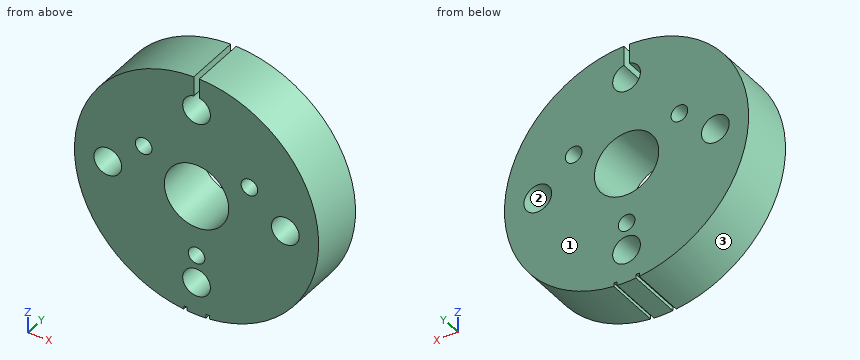
Autodesk Inventor part; units mm, degrees
ref_plane "YZ Plane" through (0, 0, 0) normal (1, 0, 0) x (0, 1, 0)
ref_plane "XZ Plane" through (0, 0, 0) normal (0, 1, 0) x (-1, 0, 0)
ref_plane "XY Plane" through (0, 0, 0) normal (0, 0, 1) x (1, 0, 0)
sketch "Эскиз1" plane through (0, 0, 0) normal (0, 1, 0) x (-1, 0, 0)
  arc A0 (-0.25, 9.2247) -> (0.25, 9.2247) centre (0, 8) ccw
  line L0 (-0.25, 10.9972) -> (-0.25, 9.2247)
  arc A1 (-0.25, 10.9972) -> (-1.1469, -10.94) centre (0, 0) ccw
  line L1 (-1.1469, -10.6297) -> (-1.1469, -10.94)
  line L2 (-0.8473, -10.6297) -> (-1.1469, -10.6297)
  line L3 (-0.8473, -10.9673) -> (-0.8473, -10.6297)
  arc A2 (-0.8473, -10.9673) -> (0.8535, -10.9668) centre (0, 0) ccw
  line L4 (0.8535, -10.6297) -> (0.8535, -10.9668)
  line L5 (1.1541, -10.6297) -> (0.8535, -10.6297)
  line L6 (1.1541, -10.9393) -> (1.1541, -10.6297)
  arc A3 (1.1541, -10.9393) -> (0.25, 10.9972) centre (0, 0) ccw
  line L7 (0.25, 9.2247) -> (0.25, 10.9972)
  circle A4 centre (8, 0) radius 1.25
  circle A5 centre (0, -8) radius 1.25
  circle A6 centre (-8, 0) radius 1.25
  circle A7 centre (0, -5.5) radius 0.75
  circle A8 centre (4.7631, 2.75) radius 0.75
  circle A9 centre (-4.7631, 2.75) radius 0.75
  circle A10 centre (0, 0) radius 2.9
  arc A11 (0.25, 9.2247) -> (-0.25, 9.2247) centre (0, 8) ccw
extrude "Выдавливание1" add sketch "Эскиз1" along normal blind 5 contours A0 L7 A3 L6 L5 L4 A2 L3 L2 L1 A1 L0
properties part number "проставка"
Could you check a few things on this model? Use its own coordinates, in mm. Face numbers are marked on the shaded views. Coordinates: 2 decimals unless noted, no trailing zeros. Write each loop counter-clockwise with the first axis right and the second up, starting at its lowest first coordinate (ties: lowest second). Pieces come first, ordered by that corner, then holes. Notation, with made-up numbers: M 65.5,24 L 116.5,24 A17 ccw 116.5,44 Z; hole C 1.25,-31.5 d11. An arc over 180 degrees is marked long. Answer as CSV lines item,"result". Start each with the question number.
1) I want a section at A-A, the plane x = -1.75. Please give me the cut outline in (y, z).
2) I want a section at C-C, the plane y = 2.25. Please give me the cut outline in (x, z).
3) I want a section at B-B, the plane z = 9.5. Please give me the cut outline in (x, y).
4) Please list where these lines run through material, in increasing order: line 1 (Z direction, x = 0, y = 2.3); line 2 (X direction, y = 4.5, z = 3.25); line 3 (Z direction, x = 8, y = 4.05). Write a range as from..to.
5) For P1, Ø2, axis at y = 4, z = -2.5, coming from the -X side; P2, Ø1.4, axis at x = -4.76, z = 2.75, coming from the -Y side; P3, Ø1, axis at x = 1.5, y = 3.5, coming from the -Z side; P4, Ø0.9, axis at y = 3.5, z = 10, coming from the -X side, each with a flat end and sliding along its axis, tell me the tip position at first contact or that it passes through.
6) We'd pull the mould along X, two halves only. Please class the marked faces 1, 2 and 3: +X half, -X half, draft (parallel to the pull), parting line (faces both ways), or undercut.
7) I want a section at D-D, the plane z = 5. Please give me the cut outline in (x, y), and give its area (3 significant figures).
Data:
1,outline,"M 0,-10.86 L 5,-10.86 L 5,-2.31 L 0,-2.31 Z; M 0,2.31 L 5,2.31 L 5,10.86 L 0,10.86 Z"
2,outline,"M -1.15,-10.94 L -1.15,-10.63 L -0.85,-10.63 L -0.85,-10.97 A11 ccw 0.85,-10.97 L 0.85,-10.63 L 1.15,-10.63 L 1.15,-10.94 A11 ccw 0.25,11 L 0.25,9.22 A1.25 cw long -0.25,9.22 L -0.25,11 A11 ccw Z; hole C -8,0 d2.5; hole C -4.76,2.75 d1.5; hole C 0,0 d5.8; hole C 0,-8 d2.5; hole C 0,-5.5 d1.5; hole C 4.76,2.75 d1.5; hole C 8,0 d2.5"
3,outline,"M -5.55,0 L -0.25,0 L -0.25,5 L -5.55,5 Z; M 0.25,0 L 5.55,0 L 5.55,5 L 0.25,5 Z"
4,line 1,"z = -11..-9.25, -6.75..-6.25, -4.75..-2.9, 2.9..6.75"
4,line 2,"x = -10.51..-5.32, -4.2..4.2, 5.32..10.51"
4,line 3,"z = -7.55..-1.25, 1.25..7.55"
5,P1,"stops at x = -10.9"
5,P2,"passes through"
5,P3,"stops at z = -10.94"
5,P4,"stops at x = -5.46"
6,face 1,"draft"
6,face 2,"undercut"
6,face 3,"-X half"
7,outline,"M -9.8,0 L 9.8,0 L 9.8,5 L -9.8,5 Z"
7,area,"98.0 mm^2"
